Autodesk Fusion 360 part; units mm, degrees
sketch "Sketch1" plane through (0, 0, 0) normal (0, 0, 1) x (1, 0, 0)
  line L0 (0, 0) -> (17, 0)
  line L1 (17, 0) -> (17, 14.1)
  line L2 (17, 14.1) -> (0, 14.1)
  line L3 (0, 14.1) -> (0, 0)
  line L4 (-2, -2) -> (19, -2)
  line L5 (19, -2) -> (19, 16)
  line L6 (19, 16) -> (-2, 16)
  line L7 (-2, 16) -> (-2, -2)
  dimension "d1" = 17
  dimension "d2" = 14.1
extrude "Extrude1" add sketch "Sketch1" along normal blind 60
fillet "Fillet1" radius 2 2 edges at (-2, -2, 30) (19, -2, 30)
Read the model definition and answer for the solid it produces. Units are mm, in the model's axes. A direction names the side the tool comes from. Round coordinates to 2 decimals unless told otherwise and drop trailing zeros. Write each loop counter-clockwise with the first axis right and the second up, starting at its lowest first coordinate (ties: lowest second). Pieces come first, ordered by that corner, then holes. Notation, with made-up numbers: (11.5, 59) - (38.5, 59) arc R20 ccw to (38.5, 83) - close; hole circle Ø11 at (47.5, -9). An arc over 180 degrees is marked (long way). Use a Markdown table: item, result.
(1) Straight lines are drawn through the part: line 1 along X through (y, z) = (6, 41); line 2 along Y through (x, z) = (7, 43.5); line 3 along X through (y, z) = (-1, 27.5). For each, find the intervals that lie inside material, in ascending order. Write a range as [from, to].
Reported:
| item | result |
|---|---|
| line 1 | [-2, 0], [17, 19] |
| line 2 | [-2, 0], [14.1, 16] |
| line 3 | [-1.73, 18.73] |
(2) The mould has two halves that part along Y. Classify faces 1 (the flat face through (0, 7, 30)), 2 (the flat face through (8, 15, 60)), 3 (the flat face through (8, -2, 30)), 4 (the flat face through (9, 14.1, 30)): released by +Y, released by -Y, zero draft, split by the parting line, or undercut.
Reported:
| item | result |
|---|---|
| face 1 | undercut |
| face 2 | zero draft |
| face 3 | released by -Y |
| face 4 | undercut |
(3) Which of the six approach directions +Z, -Z, +X, -X, +Y, -Y give full straight-line access (tool end or side, diameter ignored) to faces 5 (the flat face through (8, 15, 0)), 6 (the flat face through (17, 7, 30))?
Reported:
| item | result |
|---|---|
| face 5 | -Z, +X, -X, +Y, -Y |
| face 6 | +Z, -Z |
(4) The part is cut by section B-B (x = 5.5). Write down the section's boundary in (y, z), then the cut area to 3 significant figures.
Reported:
| item | result |
|---|---|
| outline | (-2, 0) - (0, 0) - (0, 60) - (-2, 60) - close; (14.1, 0) - (16, 0) - (16, 60) - (14.1, 60) - close |
| area | 234 mm2 |
(5) The part is cut by section A-A (y = 11). Write down the section's boundary in (x, z).
Reported:
| item | result |
|---|---|
| outline | (-2, 0) - (0, 0) - (0, 60) - (-2, 60) - close; (17, 0) - (19, 0) - (19, 60) - (17, 60) - close |
(6) The part is cut by section C-C (z = 13.5). Write down the section's boundary in (x, y).
Reported:
| item | result |
|---|---|
| outline | (-2, 0) arc R2 ccw to (0, -2) - (17, -2) arc R2 ccw to (19, 0) - (19, 16) - (-2, 16) - close; hole (0, 0) - (17, 0) - (17, 14.1) - (0, 14.1) - close |
